Drawing for the job (mm, zero at the part's lowest x, y, z). A direction names the side the tool comes from. Coordinates: 2 decimals unless noted, no trailing zeros. Write each loop counter-clockwise with the first axis right and the second up, starting at its lowest first coordinate (ties: lowest second). Pieces come first, ordered by that corner, then holes. Notation, with made-up numbers: M 19.25,-20 L 44.25,-20 A31 ccw 44.25,17 Z; hole C 77.25,83 d1. An arc over 180 degrees is marked long. Put each result on its own line as item: value. Start each with the question number.
Q1. Cut at B-B (y = 9.75). Write the cut outline in (x, z) (1 decimal).
Q2. Cut at D-D (z = 4.85). Write the cut outline in (x, y).
Q3. Cut at C-C (y = 19.5). Write the cut outline in (x, z) (1 decimal), then the cut area to 3 significant figures.
Q4. Drill centre lines: line 1 along Y through (x, z) = (1.55, 1.05); line 2 along X through (y, z) = (23.5, 2.05); line 3 along X through (y, z) = (12, 0.5) (1 decimal). Where is each one in solid material? Low to high.
Q5. Pull direction X, two halves, no side cores. Call the marked faces 3, 4, 5 and 6: pulls with the +X half, pulls with the -X half, needs draft (parallel to the pull), parting line crosses it, or undercut.
Q6. Which spindle directions (+Z, -Z, +X, -X, +Y, -Y) get a long thin tool onto all of the face, cutting with end or side? Do the marked faces 1 and 2. Say none if no direction does.
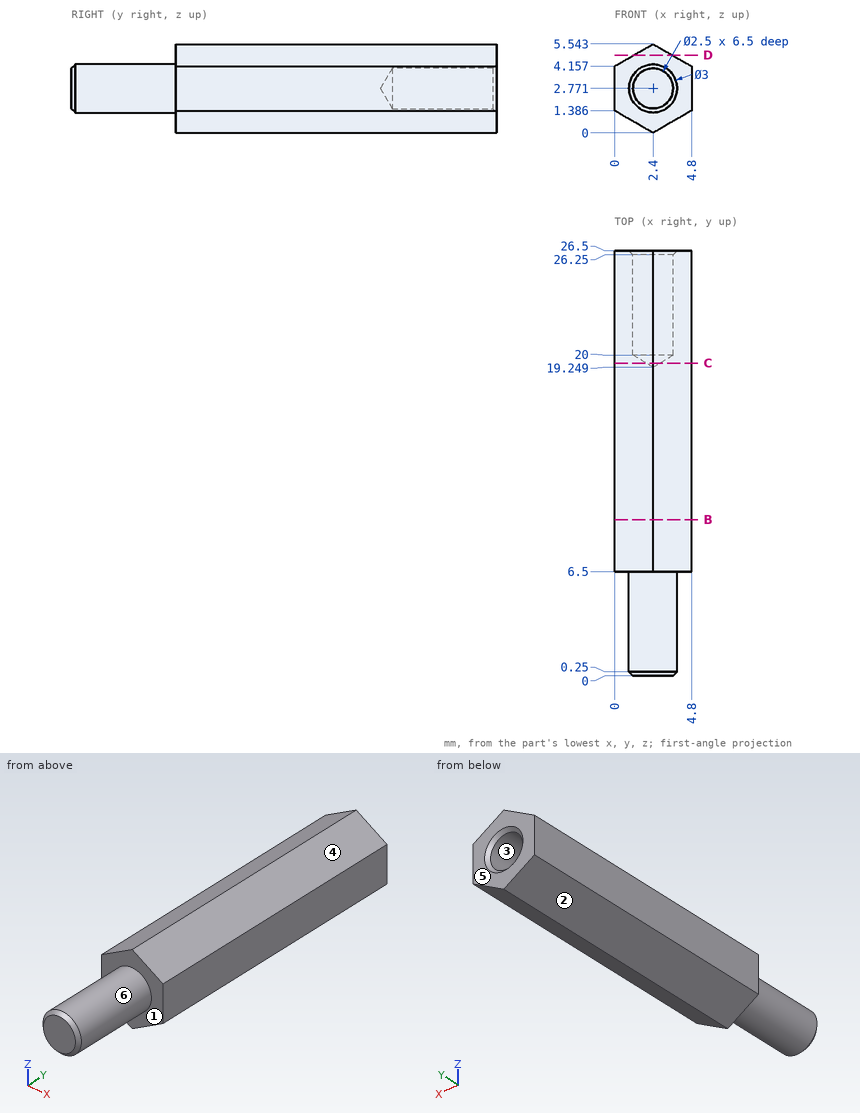
Computed values:
1. outline: M 0,1.4 L 2.4,0 L 4.8,1.4 L 4.8,4.2 L 2.4,5.5 L 0,4.2 Z
2. outline: M 1.2,6.5 L 3.6,6.5 L 3.6,26.5 L 1.2,26.5 Z
3. outline: M 0,1.4 L 2.4,0 L 4.8,1.4 L 4.8,4.2 L 2.4,5.5 L 0,4.2 Z; hole C 2.4,2.8 d0.8
3. area: 19.4 mm2
4. line 1: 6.5 to 26.5
4. line 2: 0 to 1.38, 3.42 to 4.8
4. line 3: 1.5 to 3.3
5. face 3: undercut
5. face 4: pulls with the +X half
5. face 5: needs draft
5. face 6: parting line crosses it
6. face 1: -Y
6. face 2: -Z, -X, +Y, -Y
